```python
from build123d import *
from OCP.BRepFilletAPI import BRepFilletAPI_MakeChamfer

# Parameters (mm, degrees)
SKETCH_1_W          = 77
SKETCH_1_H          = 21.5
EXTRUDE_1_DEPTH     = 15.1
CHAMFER_1_SIZE      = 7.3
CHAMFER_1_SIZE2     = 2
CUT_EXTRUDE_1_DEPTH = 47.610192018
CUT_EXTRUDE_START   = -3.8
SKETCH_3_R          = 9.15
CUT_EXTRUDE_2_DEPTH = 69.4
SKETCH_4_W          = 67.4
SKETCH_4_H          = 8
SKETCH_4_W_2        = 2.4
SKETCH_4_H_2        = 3.7
CUT_EXTRUDE_3_DEPTH = 43.729644302


with BuildPart() as part:
    # Эскиз1 → Бобышка-Вытянуть1 (new body)
    with BuildSketch(Plane(origin=(0, 0, 0), x_dir=(1, 0, 0), z_dir=(0, 1, 0))):
        Rectangle(SKETCH_1_W, SKETCH_1_H)
    extrude(amount=EXTRUDE_1_DEPTH)

    # Фаска1: one chamfer whose edges measure the first distance from different faces: ONE call of the kernel's chamfer builder (chamfer() names one face for all edges)
    chamfer_1_edges_1 = [part.edges().sort_by_distance(p)[0] for p in [
        (0, 15.1, 10.75),
    ]]
    chamfer_1_side_1 = [part.faces().sort_by_distance(p)[0] for p in [
        (0, 7.55, 10.75),
    ]]
    chamfer_1_edges_2 = [part.edges().sort_by_distance(p)[0] for p in [
        (0, 15.1, -10.75),
    ]]
    chamfer_1_side_2 = [part.faces().sort_by_distance(p)[0] for p in [
        (0, 7.55, -10.75),
    ]]
    chamfer_1 = BRepFilletAPI_MakeChamfer(part.part.solid().wrapped)
    for e in chamfer_1_edges_1:
        chamfer_1.Add(CHAMFER_1_SIZE, CHAMFER_1_SIZE2, e.wrapped, chamfer_1_side_1[0].wrapped)  # the first distance lies on this face
    for e in chamfer_1_edges_2:
        chamfer_1.Add(CHAMFER_1_SIZE, CHAMFER_1_SIZE2, e.wrapped, chamfer_1_side_2[0].wrapped)  # the first distance lies on this face
    add(Compound.cast(chamfer_1.Shape()), mode=Mode.REPLACE)

    # Эскиз2 → Вырез-Вытянуть1 (cut, through all)
    with BuildSketch(Plane.XY.offset(10.75)):
        with BuildLine():
            Line((-34.7, 15.1), (34.7, 15.1))
            Line((34.7, 15.1), (34.7, 9.3))
            ThreePointArc((34.7, 9.3), (34.114213562, 7.885786438), (32.7, 7.3))
            Line((32.7, 7.3), (-32.7, 7.3))
            ThreePointArc((-32.7, 7.3), (-34.114213562, 7.885786438), (-34.7, 9.3))
            Line((-34.7, 9.3), (-34.7, 15.1))
        make_face()
    extrude(amount=-CUT_EXTRUDE_1_DEPTH, mode=Mode.SUBTRACT)

    # Эскиз3 → Вырез-Вытянуть2 (cut)
    with BuildSketch(Plane(origin=(38.5, 0, 0), x_dir=(0, 0, -1), z_dir=(1, 0, 0)).offset(CUT_EXTRUDE_START)):
        with Locations((0, 9.25)):
            Circle(SKETCH_3_R)
    extrude(amount=-CUT_EXTRUDE_2_DEPTH, mode=Mode.SUBTRACT)

    # Эскиз4 → Вырез-Вытянуть3 (cut, through all)
    with BuildSketch(Plane.XZ):
        Rectangle(SKETCH_4_W, SKETCH_4_H)
        with Locations((-37.3, 0)):
            Rectangle(SKETCH_4_W_2, SKETCH_4_H_2)
        with Locations((37.3, 0)):
            Rectangle(SKETCH_4_W_2, SKETCH_4_H_2)
    extrude(amount=-CUT_EXTRUDE_3_DEPTH, mode=Mode.SUBTRACT)


solid = part.part
```
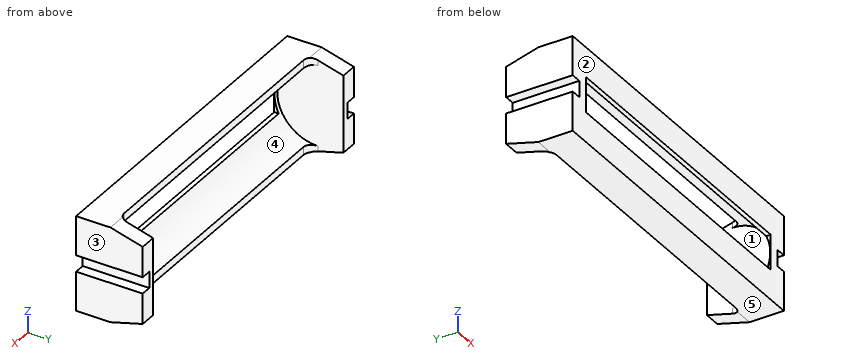
Check sheet for the modelled part. Datum: model origin and axes. Units: mm. Face numbers are marked on the shaded views. A direction names the side the tool comes from. Round coordinates to 2 decimals unless told otherwise and drop trailing zeros. Order: outer loops, then holes, each group sorted by start corner. A loop starts at its lowest first (then second) coordinate and runs counter-clockwise, first axis right, second up. Notation, with made-up numbers: (37, 0) - (45, 0) arc R13 cw to (45, 20) - close; hole circle Ø5 at (44.5, -7.5). An arc over 180 degrees is marked (long way). Write item = value, one per line.
Q1. Draft check along Z on the marked faces 3, 4 and 5. Enter one of: pulls with the +Z half, pulls with the -Z half, needs draft (parallel to the pull), parting line crosses it, or undercut.
Computed:
face_3 = needs draft
face_4 = undercut
face_5 = pulls with the -Z half
Q2. Section check C-C (y = 13.75). Record the boundary of the cut face in (x, z), and give its area (3 significant figures).
Computed:
outline = (-38.5, -9.12) - (-34.7, -9.12) - (-34.7, 9.12) - (-38.5, 9.12) - (-38.5, 1.85) - (-36.1, 1.85) - (-36.1, -1.85) - (-38.5, -1.85) - close; (34.7, -9.12) - (38.5, -9.12) - (38.5, -1.85) - (36.1, -1.85) - (36.1, 1.85) - (38.5, 1.85) - (38.5, 9.12) - (34.7, 9.12) - close
area = 121 mm^2
Q3. Section check A-A (x = 24). Record the boundary of the cut face in (y, z), and give its area (3 significant figures).
Computed:
outline = (0, -10.75) - (7.3, -10.75) - (7.3, -8.94) arc R9.15 cw to (1.02, -4) - (0, -4) - close; (0, 4) - (1.02, 4) arc R9.15 cw to (7.3, 8.94) - (7.3, 10.75) - (0, 10.75) - close
area = 57.6 mm^2
Q4. Section check D-D (y = 3.25). Record the boundary of the cut face in (x, z), and give its area (3 significant figures).
Computed:
outline = (-38.5, -10.75) - (38.5, -10.75) - (38.5, -1.85) - (36.1, -1.85) - (36.1, 1.85) - (38.5, 1.85) - (38.5, 10.75) - (-38.5, 10.75) - (-38.5, 1.85) - (-36.1, 1.85) - (-36.1, -1.85) - (-38.5, -1.85) - close; hole (-34.7, -6.91) - (34.7, -6.91) - (34.7, 6.91) - (-34.7, 6.91) - close
area = 679 mm^2
Q5. Tool access check on the marked faces 1 and 2. Record the directions out of +Z, -Z, +X, -X, +Y, -Y that give a thin tool (end or side, any length) a straight path to the whole face; none if there is none.
Computed:
face_1 = +Y
face_2 = +Z, -Z, +X, -X, -Y
Q6. Section check B-B (z = 0). Record the boundary of the cut face in (x, y).
Computed:
outline = (-36.1, 0) - (-33.7, 0) - (-33.7, 0.1) - (-34.7, 0.1) - (-34.7, 15.1) - (-36.1, 15.1) - close; (33.7, 0) - (36.1, 0) - (36.1, 15.1) - (34.7, 15.1) - (34.7, 0.1) - (33.7, 0.1) - close
Q7. Go/stop test with flat-tipped pins: pin 1 (1.1 mm diameter, centred on y = 6, z = 0, fed in from -X); pin 2 (1.9 mm diameter, centred on x = 37.5, y = 10, fed in from +Z); pin 3 (0.5 mm diameter, centred on x = 8, z = 9.5, fed in from +Y). Record where each tip stops, or that it passes through.
Computed:
pin_1 = -36.1
pin_2 = 10.41
pin_3 = 7.3
Q8. Thickness scan on line 1 along X through (y, z) = (14, 4); line 2 along X through (y, z) = (14.25, 1); line 3 along Z through (x, y) = (-29, 0.5). Record the ranges inside material, lowest first.
Computed:
line_1 = -38.5 to -34.7, 34.7 to 38.5
line_2 = -36.1 to -34.7, 34.7 to 36.1
line_3 = -10.75 to -4, 4 to 10.75
